from build123d import *

# Parameters (mm, degrees)
SKETCH2_R           = 3.175
BOSS_EXTRUDE1_DEPTH = 44.45
CHAMFER1_SIZE       = 0.9525
CUT_EXTRUDE1_DEPTH  = 3.048
SKETCH8_R           = 2.749630657
CUT_EXTRUDE2_DEPTH  = 1.27
CUT_EXTRUDE2_DRAFT  = -45


with BuildPart() as part:
    # Sketch2 → Boss-Extrude1 (new body)
    with BuildSketch(Plane(origin=(22.225, 0, 0), x_dir=(0, 0, -1), z_dir=(1, 0, 0))):
        Circle(SKETCH2_R)
    extrude(amount=-BOSS_EXTRUDE1_DEPTH)

    # Chamfer1
    chamfer1_edges = [part.edges().sort_by_distance(p)[0] for p in [
        (22.225, 0, 3.175),
    ]]
    chamfer(chamfer1_edges, length=CHAMFER1_SIZE)

    # Sketch6 → Revolve1 (revolve)
    with BuildSketch(Plane.XY):
        Polygon((-27.94, 4.7625), (-28.575, 4.1275), (-28.575, 0), (-22.225, 0), (-22.225, 4.445), (-22.5425, 4.7625), align=None)
    revolve(axis=Axis((-22.225, 0, 0), (-1, 0, 0)))

    # Sketch4 → Cut-Extrude1 (cut)
    with BuildSketch(Plane(origin=(-28.575, 0, 0), x_dir=(0, 0, -1), z_dir=(1, 0, 0))):
        Polygon((0, 2.749630657), (-2.38125, 1.374815329), (-2.38125, -1.374815329), (0, -2.749630657), (2.38125, -1.374815329), (2.38125, 1.374815329), align=None)
    extrude(amount=CUT_EXTRUDE1_DEPTH, mode=Mode.SUBTRACT)


with BuildPart() as cut_extrude2_tool:
    # Sketch8 → Cut-Extrude2 (with draft: the straight prism first)
    with BuildSketch(Plane.ZY.offset(28.575)):
        Circle(SKETCH8_R)
    extrude(amount=-CUT_EXTRUDE2_DEPTH)
    # Cut-Extrude2: the draft: its side faces are tilted about the plane it starts from
    cut_extrude2_sides = [cut_extrude2_tool.faces().sort_by_distance(p)[0] for p in [
        (-27.94, 0, -2.749630657),
    ]]
    draft(cut_extrude2_sides, Plane.ZY.offset(28.575), CUT_EXTRUDE2_DRAFT)


with BuildPart() as part_1:
    add(part.part)

    # Cut-Extrude2: cut by cut_extrude2_tool
    add(cut_extrude2_tool.part, mode=Mode.SUBTRACT)


solid = part_1.part
CAD build for the part. Positions are in the model's coordinates, mm. A direction names the side the tool comes from. Coordinates: 2 decimals unless noted, no trailing zeros. Order: outer loops, then holes, each group sorted by start corner. A loop starts at its lowest first (then second) coordinate and runs counter-clockwise, first axis right, second up.
Item 1: Band-saw the part on B-B on x = -21. List the corners of the cut face in (y, z) (3 decimals), plus the area to 3 significant figures.
Check sheet entries:
outline: circle Ø6.35 at (0, 0)
area: 31.7 mm2
Item 2: 3-axis set-ups, long thin cutter, end or side, ignore diameter. For faces 1 (the face through (-25.28, -3.78, 2.9)), 2 (the face through (-28.39, -2.21, -1.3)): which of +Z, -Z, +X, -X, +Y, -Y reach the whole face in a straight line?
Check sheet entries:
face 1: +X, -X
face 2: -X
Item 3: Band-saw the part on A-A on y = 0. List the corners of the cut face in (x, z) (1 decimal), plus the area to 3 significant figures.
Check sheet entries:
outline: (-28.6, -4.1) - (-27.9, -4.8) - (-22.5, -4.8) - (-22.2, -4.4) - (-22.2, -3.2) - (21.3, -3.2) - (22.2, -2.2) - (22.2, 2.2) - (21.3, 3.2) - (-22.2, 3.2) - (-22.2, 4.4) - (-22.5, 4.8) - (-27.9, 4.8) - (-28.6, 4.1) - (-28.6, 2.7) - (-28.2, 2.4) - (-25.5, 2.4) - (-25.5, -2.4) - (-28.2, -2.4) - (-28.6, -2.7) - close
area: 327 mm2
Item 4: Two-plate mould, pull along Y, no slides. Class faces 3 (the face through (-28.39, 2.21, 1.3)), 4 (the face through (-0.17, -3.1, 0.69)), 5 (the face through (-22.225, -2, 3)): +Y half, -Y half, draft (parallel to the pull), parting line (faces both ways), or undercut.
Check sheet entries:
face 3: undercut
face 4: parting line
face 5: draft
Item 5: Pin check, flat tips, straight feed: pin 1 Ø5 at (x, y) = (-5.5, 0.5) entering from +Z (3 decimals); pin 2 Ø5 at (x, z) = (7, -0.5) entering from -Y (3 decimals); pin 3 Ø4 at (y, z) = (0.5, 1) entering from -X (3 decimals); pin 4 Ø3 at (x, y) = (-14, -3.5) entering from -Z. Stop position of each tip, or through.
Check sheet entries:
pin 1: stops at z = 3.175
pin 2: stops at y = -3.175
pin 3: stops at x = -28.575
pin 4: stops at z = -2.47
Item 6: Drill centre lines: L1, parallel to Y at x = -16, z = 0.25; L2, parallel to X at y = -1, z = 0.75 (3 decimals); L3, parallel to X at y = 1, z = -3.75 (3 decimals). Where is each one in solid material? Low to high.
Check sheet entries:
L1: y = -3.17 to 3.17
L2: x = -25.527 to 22.225
L3: x = -28.575 to -22.225
